Design review of the part built by this model. Coordinates are the model's own, in mm. Face numbers are marked on the shaded views. A direction names the side the tool comes from. Coordinates: 2 decimals unless noted, no trailing zeros. Loops run counter-clockwise (first coordinate to the right, second up) from the corner with the lowest first, then second, coordinate; pieces in that order, holes last. Notation, with made-up numbers: M 72.5,16.25 L 109.5,16.25 A22 ccw 109.5,29.25 Z; hole C 68.5,-28 d4. An arc over 180 degrees is marked long. Answer as CSV lines item,"result". Start each with the question number.
from build123d import *

# Parameters (mm, degrees)
F0_W      = 42
F0_H      = 42
F1_DEPTH  = 6
F2_SIZE   = 7.5
F4_DEPTH  = 12
F5_SIZE   = 5
F7_DEPTH  = 13
F8_R      = 11
F9_DEPTH  = 2
F10_R     = 2.5
F11_DEPTH = 22
F12_W     = 5.2537292178
F12_H     = 0.9334036984
F13_DEPTH = 22
F14_R     = 1.5
F15_DEPTH = 37.001
F16_W     = 16
F16_H     = 11
F17_DEPTH = 6


with BuildPart() as f1:
    # F0 (on Top) → F1 (new body, symmetric)
    with BuildSketch(Plane.XY):
        Rectangle(F0_W, F0_H)
    extrude(amount=F1_DEPTH, both=True)

    # F2
    f2_edges = [f1.edges().sort_by_distance(p)[0] for p in [
        (21, 21, 0),
        (-21, 21, 0),
        (-21, -21, 0),
        (21, -21, 0),
    ]]
    chamfer(f2_edges, length=F2_SIZE)

    # F3 (on face) → F4 (join)
    with BuildSketch(Plane.XY.offset(6)):
        Polygon((13.5, 21), (-13.5, 21), (-21, 13.5), (-21, -13.5), (-13.5, -21), (13.5, -21), (21, -13.5), (21, 13.5), align=None)
        Polygon((21, 21), (13.5, 21), (21, 13.5), align=None)
        Polygon((-13.5, 21), (-21, 21), (-21, 13.5), align=None)
        Polygon((-13.5, -21), (-21, -13.5), (-21, -21), align=None)
        Polygon((21, -21), (21, -13.5), (13.5, -21), align=None)
    extrude(amount=F4_DEPTH)

    # F5
    f5_edges = [f1.edges().sort_by_distance(p)[0] for p in [
        (21, -21, 12),
        (-21, -21, 12),
        (-21, 21, 12),
        (21, 21, 12),
    ]]
    chamfer(f5_edges, length=F5_SIZE)

    # F6 (on face) → F7 (join)
    with BuildSketch(Plane(origin=(0, 0, -6), x_dir=(1, 0, 0), z_dir=(0, 0, -1))):
        Polygon((21, -16), (21, 16), (16, 21), (-16, 21), (-21, 16), (-21, -16), (-16, -21), (16, -21), align=None)
    extrude(amount=F7_DEPTH)

    # F8 (on face) → F9 (join)
    with BuildSketch(Plane.XY.offset(18)):
        Circle(F8_R)
    extrude(amount=F9_DEPTH)

    # F10 (on face) → F11 (join)
    with BuildSketch(Plane.XY.offset(20)):
        Circle(F10_R)
    extrude(amount=F11_DEPTH)

    # F12 (on face) → F13 (cut)
    with BuildSketch(Plane.XY.offset(42)):
        with Locations((-0.0065014465, 2.4667018492)):
            Rectangle(F12_W, F12_H)
    extrude(amount=-F13_DEPTH, mode=Mode.SUBTRACT)

    # F14 (on face) → F15 (cut, through all)
    with BuildSketch(Plane.XY.offset(18)):
        with Locations((-15.5, 15.5)):
            Circle(F14_R)
        with Locations((15.5, 15.5)):
            Circle(F14_R)
        with Locations((-15.5, -15.5)):
            Circle(F14_R)
        with Locations((15.5, -15.5)):
            Circle(F14_R)
    extrude(amount=-F15_DEPTH, mode=Mode.SUBTRACT)

    # F16 (on face) → F17 (join)
    with BuildSketch(Plane(origin=(0, 21, 0), x_dir=(-1, 0, 0), z_dir=(0, 1, 0))):
        with Locations((0, -13.5)):
            Rectangle(F16_W, F16_H)
    extrude(amount=F17_DEPTH)


solid = f1.part
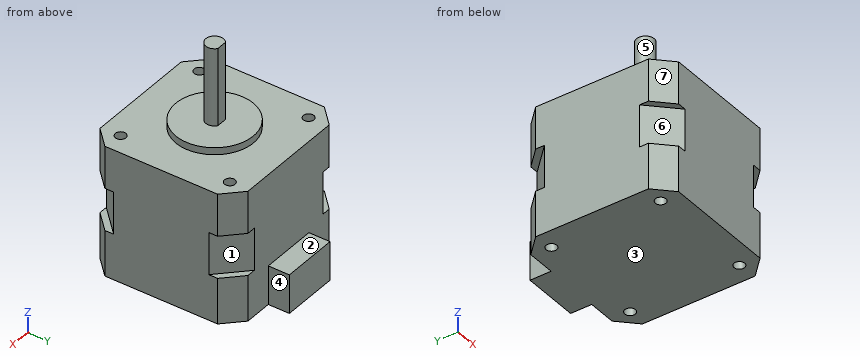
Item 1: For the marked faces 4, 5, 6 and 7, list the 3-axis set-ups (+Z, -Z, +X, -X, +Y, -Y) from which the entire face can be reached by the end or side of a thin tool; tool diameter is ignored.
Item 2: Mouldability with a two-part tool opening along Z and no side actions: class the marked faces 1, 2 and 3 as released by +Z, released by -Z, zero draft, split by the parting line, or undercut.
Item 3: For pin 1 (5 mm diameter, centred on y = 24.5, z = -16, fed in from -X); pin 2 (5 mm diameter, centred on y = 24, z = -11.5, fed in from +X); pin 3 (2 mm diameter, centred on x = 16.5, y = -18.5, fed in from +Z); pin 4 (2.5 mm diameter, centred on x = -15.5, y = -15.5, fed in from +Z), all flat-tipped, find the tip position at first contact; note any pin that passes through.
Item 4: Add section A-A (z = -9). Give the boundary of the cut face in (x, y).
Item 5: For line 1 along Y through (x, z) = (14.5, 5); line 2 along X through (y, z) = (-15, -7); line 3 along X through (y, z) = (-15, 4), list the stretches that pass through material, from the lowest coordinate up. Write a range as from..to.
Item 6: Add section D-D (z = 31.5). Give the boundary of the cut face in (x, y), plus the area to 3 significant figures.
Item 7: Add section C-C (y = 0). Give the boundary of the cut face in (x, z), plus the area to 3 significant figures.
Item 8: Add section B-B (x = -18). Give the boundary of the cut face in (y, z), plus the area to 3 significant figures.
Response:
1,face 4,"+Z, -Z, +X, +Y"
1,face 5,"+Z"
1,face 6,"-X, -Y"
1,face 7,"+Z, -Z, -X, -Y"
2,face 1,"undercut"
2,face 2,"released by +Z"
2,face 3,"released by -Z"
3,pin 1,"x = -8"
3,pin 2,"x = 8"
3,pin 3,"z = 18"
3,pin 4,"through"
4,outline,"M -21,-16 L -16,-21 L 16,-21 L 21,-16 L 21,16 L 16,21 L 8,21 L 8,27 L -8,27 L -8,21 L -16,21 L -21,16 Z; hole C -15.5,-15.5 d3; hole C -15.5,15.5 d3; hole C 15.5,-15.5 d3; hole C 15.5,15.5 d3"
5,line 1,"-20..-16.62, -14.38..14.38, 16.62..20"
5,line 2,"-21..-16.91, -14.09..14.09, 16.91..21"
5,line 3,"-19.5..-16.91, -14.09..14.09, 16.91..19.5"
6,outline,"M -1.5,2 A2.5 ccw long 1.5,2 Z"
6,area,"18.6 mm²"
7,outline,"M -21,-19 L 21,-19 L 21,18 L 11,18 L 11,20 L 2.5,20 L 2.5,42 L -2.5,42 L -2.5,20 L -11,20 L -11,18 L -21,18 Z"
7,area,"1,710 mm²"
8,outline,"M -19,-19 L 19,-19 L 19,-6 L 16.5,-6 L 16.5,6 L 19,6 L 19,18 L -19,18 L -19,6 L -16.5,6 L -16.5,-6 L -19,-6 Z"
8,area,"1,350 mm²"
